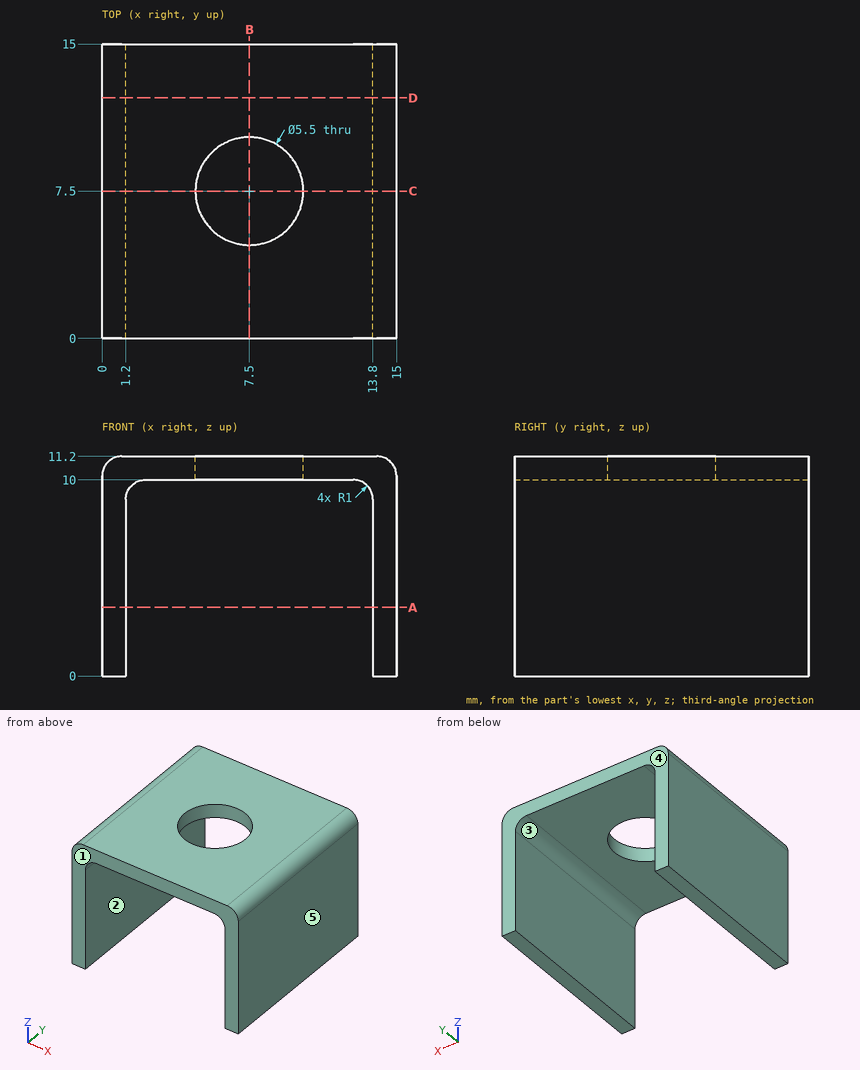
Design review of the part shown in the three views and the two pictorial views. Dimensions are in mm from the part's minimum x, y and z. A direction names the side the tool comes from. Coordinates: 2 decimals unless noted, no trailing zeros. Loops run counter-clockwise (first coordinate to the right, second up) from the corner with the lowest first, then second, coordinate; pieces in that order, holes last. Notation, with made-up numbers: (80.5, 12) - (84.5, 12) arc R22 ccw to (84.5, 43) - close; hole circle Ø5 at (-20.75, 56). An arc over 180 degrees is marked (long way). Use a Markdown table: item, result. Add a question column.
Item 1: We need section A-A (z = 3.5). Give the boundary of the cut face in (x, y).
Item 2: Insertion check: pin 1 Ø4 at (x, y) = (3.5, 6.5) entering from -Z; pin 2 Ø3 at (x, y) = (5.5, 4.5) entering from -Z; pin 3 Ø1.5 at (x, z) = (12, 4.5) entering from -Y. Each pin has a flat end and moves straight along its axis. Give the tip position at first contact, or say it passes through.
Item 3: We need section B-B (x = 7.5). Give the boundary of the cut face in (y, z), and give its area (3 significant figures).
Item 4: For line 1 (Y direction, x = 7.5, z = 10.55); line 2 (X direction, y = 8.75, z = 1.5); line 3 (Z direction, x = 11, y = 9.25), list the stretches that pass through material, from the lowest coordinate up.
Item 5: We need section D-D (y = 12.25). Give the boundary of the cut face in (x, z), and give its area (3 significant figures).
Item 6: Mouldability with a two-part tool opening along X and no side actions: class the marked faces 3, 4 and 5 as pulls with the +X half, pulls with the -X half, needs draft (parallel to the pull), parting line crosses it, or undercut.
Item 7: We need section C-C (y = 7.5). Give the boundary of the cut face in (x, z).
Item 8: Tool access review of the marked faces 1 and 2: name each direction out of +Z, -Z, +X, -X, +Y, -Y from which nothing blocks a thin tool from reaching the whole face with its end or side.
Results list:
| question | item | result |
|---|---|---|
| 1 | outline | (0, 0) - (1.2, 0) - (1.2, 15) - (0, 15) - close; (13.8, 0) - (15, 0) - (15, 15) - (13.8, 15) - close |
| 2 | pin 1 | stops at z = 9.71 |
| 2 | pin 2 | stops at z = 10 |
| 2 | pin 3 | passes through |
| 3 | outline | (0, 10) - (4.75, 10) - (4.75, 11.2) - (0, 11.2) - close; (10.25, 10) - (15, 10) - (15, 11.2) - (10.25, 11.2) - close |
| 3 | area | 11.4 mm^2 |
| 4 | line 1 | y = 0 to 4.75, 10.25 to 15 |
| 4 | line 2 | x = 0 to 1.2, 13.8 to 15 |
| 4 | line 3 | z = 10 to 11.2 |
| 5 | outline | (0, 0) - (1.2, 0) - (1.2, 9) arc R1 cw to (2.2, 10) - (12.8, 10) arc R1 cw to (13.8, 9) - (13.8, 0) - (15, 0) - (15, 10.2) arc R1 ccw to (14, 11.2) - (1, 11.2) arc R1 ccw to (0, 10.2) - close |
| 5 | area | 42.0 mm^2 |
| 6 | face 3 | undercut |
| 6 | face 4 | needs draft |
| 6 | face 5 | pulls with the +X half |
| 7 | outline | (0, 0) - (1.2, 0) - (1.2, 9) arc R1 cw to (2.2, 10) - (4.75, 10) - (4.75, 11.2) - (1, 11.2) arc R1 ccw to (0, 10.2) - close; (10.25, 10) - (12.8, 10) arc R1 cw to (13.8, 9) - (13.8, 0) - (15, 0) - (15, 10.2) arc R1 ccw to (14, 11.2) - (10.25, 11.2) - close |
| 8 | face 1 | +Z, -Z, +X, -X, -Y |
| 8 | face 2 | -Z, +Y, -Y |
